```python
from build123d import *

# Parameters (mm, degrees)
BOSS_EXTRUDE1_DEPTH   = 227
CUT_EXTRUDE1_DEPTH    = 257.229581821
SKETCH3_W             = 10
SKETCH3_H             = 15.5
CUT_EXTRUDE2_DEPTH    = 234.473879022
SKETCH4_W             = 15.5
SKETCH4_H             = 10
CUT_EXTRUDE3_DEPTH    = 252.639093083
FILLET3_R             = 1.5
BOSS_EXTRUDE3_DEPTH   = 1.5
BOSS_EXTRUDE4_DEPTH   = 1.5
SKETCH9_W             = 26
SKETCH9_H             = 12
BOSS_EXTRUDE5_DEPTH   = 1.5
SKETCH10_W            = 12
SKETCH10_H            = 26
BOSS_EXTRUDE6_DEPTH   = 1.5
FILLET7_R             = 5
SKETCH11_R            = 2
CUT_EXTRUDE4_DEPTH    = 10
SKETCH12_R            = 2
CUT_EXTRUDE5_DEPTH    = 10
FILLET8_R             = 0.2
F_3_0MM_DOWEL_HOLE1_D = 3
F_3_0MM_DOWEL_HOLE2_D = 3


with BuildPart() as part:
    # Sketch1 → Boss-Extrude1 (new body)
    with BuildSketch(Plane.XY):
        Polygon((5.710530524, 107.230570717), (35.710530524, 107.230570717), (35.710530524, 97.694605712), (39.660530524, 97.694605712), (42.571762587, 100.605837775), (44.621762586, 98.555837776), (41.710530523, 95.644605712), (41.710530523, 91.694605712), (51.246495528, 91.694605712), (51.246495528, 61.694605712), align=None)
    extrude(amount=BOSS_EXTRUDE1_DEPTH)

    # Sketch2 → Cut-Extrude1 (cut, through all)
    with BuildSketch(Plane(origin=(0, 0, 0), x_dir=(-1, 0, 0), z_dir=(0, 0, -1))):
        Polygon((-45.246495528, 88.994605712), (-45.246495528, 80.994605712), (-43.746495528, 80.994605712), (-43.746495528, 88.994605712), (-39.660530524, 88.994605712), (-33.010530524, 95.644605712), (-33.010530524, 99.730570717), (-25.010530524, 99.730570717), (-25.010530524, 101.230570717), (-33.010530524, 101.230570717), (-33.010530524, 106.694605712), (-36.710530524, 106.694605712), (-36.710530524, 108.694605712), (27.289469476, 108.694605712), (-52.710530523, 28.694605712), (-52.710530523, 92.694605712), (-50.710530523, 92.694605712), (-50.710530523, 88.994605712), align=None)
    extrude(amount=-CUT_EXTRUDE1_DEPTH, mode=Mode.SUBTRACT)

    # Sketch3 → Cut-Extrude2 (cut, through all)
    with BuildSketch(Plane(origin=(0, 101.230570717, 0), x_dir=(1, 0, 0), z_dir=(0, 1, 0))):
        with Locations((28.010530524, -5.75)):
            Rectangle(SKETCH3_W, SKETCH3_H)
        with Locations((28.010530524, -221.25)):
            Rectangle(SKETCH3_W, SKETCH3_H)
        with BuildLine():
            Line((31.010530524, -28.5), (31.010530524, -198.5))
            ThreePointArc((31.010530524, -198.5), (29.010530524, -200.5), (27.010530524, -198.5))
            Line((27.010530524, -198.5), (27.010530524, -28.5))
            ThreePointArc((27.010530524, -28.5), (29.010530524, -26.5), (31.010530524, -28.5))
        make_face()
    extrude(amount=-CUT_EXTRUDE2_DEPTH, mode=Mode.SUBTRACT)

    # Sketch4 → Cut-Extrude3 (cut, through all)
    with BuildSketch(Plane(origin=(45.246495528, 0, 0), x_dir=(0, 0, -1), z_dir=(1, 0, 0))):
        with Locations((-221.25, 83.994605712)):
            Rectangle(SKETCH4_W, SKETCH4_H)
        with Locations((-5.75, 83.994605712)):
            Rectangle(SKETCH4_W, SKETCH4_H)
        with BuildLine():
            Line((-198.5, 86.994605712), (-28.5, 86.994605712))
            ThreePointArc((-28.5, 86.994605712), (-26.5, 84.994605712), (-28.5, 82.994605712))
            Line((-28.5, 82.994605712), (-198.5, 82.994605712))
            ThreePointArc((-198.5, 82.994605712), (-200.5, 84.994605712), (-198.5, 86.994605712))
        make_face()
    extrude(amount=-CUT_EXTRUDE3_DEPTH, mode=Mode.SUBTRACT)

    # Fillet3
    # the kernel refuses this fillet: 1.5 mm, written as the material it takes off along each edge
    with BuildSketch(Plane(origin=(44.621762586, 98.555837776, -3.75), x_dir=(-0.7071067811865522, -0.7071067811865428, 0), z_dir=(0, 0, 1)), Plane(origin=(42.571762587, 100.605837775, -3.75), x_dir=(0.7071067811865476, -0.7071067811865476, 0), z_dir=(0, 0, 1))) as fillet3_piece_1:
        with BuildLine():
            CenterArc((FILLET3_R, -FILLET3_R), FILLET3_R, 90, 90)
            Line((0, -FILLET3_R), (0, 0))
            Line((0, 0), (FILLET3_R, 0))
        make_face()
    extrude(amount=234.5, mode=Mode.SUBTRACT)

    # Sketch6 → Boss-Extrude3 (add)
    with BuildSketch(Plane(origin=(0, 0, 13.5), x_dir=(-1, 0, 0), z_dir=(0, 0, -1))):
        Polygon((-45.246495528, 90.194605712), (-45.246495528, 65.230570717), (-33.246495528, 65.230570717), (-33.246495528, 89.230570717), (-9.246495528, 89.230570717), (-9.246495528, 101.230570717), (-34.210530524, 101.230570717), (-34.210530524, 96.230570717), (-40.246495528, 90.194605712), align=None)
    extrude(amount=BOSS_EXTRUDE3_DEPTH)

    # Sketch7 → Boss-Extrude4 (add)
    with BuildSketch(Plane.XY.offset(213.5)):
        Polygon((9.246495528, 101.230570717), (34.210530524, 101.230570717), (34.210530524, 96.230570717), (40.246495528, 90.194605712), (45.246495528, 90.194605712), (45.246495528, 65.230570717), (33.246495528, 65.230570717), (33.246495528, 89.230570717), (9.246495528, 89.230570717), align=None)
    extrude(amount=BOSS_EXTRUDE4_DEPTH)

    # Sketch9 → Boss-Extrude5 (add)
    with BuildSketch(Plane(origin=(0, 101.230570717, 0), x_dir=(1, 0, 0), z_dir=(0, 1, 0))):
        with Locations((22.246495528, -209)):
            Rectangle(SKETCH9_W, SKETCH9_H)
        with Locations((22.246495528, -18)):
            Rectangle(SKETCH9_W, SKETCH9_H)
    extrude(amount=-BOSS_EXTRUDE5_DEPTH)

    # Sketch10 → Boss-Extrude6 (add)
    with BuildSketch(Plane(origin=(45.246495528, 0, 0), x_dir=(0, 0, -1), z_dir=(1, 0, 0))):
        with Locations((-209, 78.230570717)):
            Rectangle(SKETCH10_W, SKETCH10_H)
        with Locations((-18, 78.230570717)):
            Rectangle(SKETCH10_W, SKETCH10_H)
    extrude(amount=-BOSS_EXTRUDE6_DEPTH)

    # Fillet7
    fillet7_edges = [part.edges().sort_by_distance(p)[0] for p in [
        (33.246495528, 65.230570717, 12.75),
        (33.246495528, 89.230570717, 12.75),
        (9.246495528, 89.230570717, 12.75),
        (9.246495528, 89.230570717, 214.25),
        (33.246495528, 89.230570717, 214.25),
        (33.246495528, 65.230570717, 214.25),
        (9.246495528, 100.480570717, 203),
        (25.010530524, 100.480570717, 203),
        (9.246495528, 100.480570717, 24),
        (25.010530524, 100.480570717, 24),
        (44.496495528, 65.230570717, 203),
        (44.496495528, 80.994605712, 203),
        (44.496495528, 65.230570717, 24),
        (44.496495528, 80.994605712, 24),
    ]]
    fillet(fillet7_edges, radius=FILLET7_R)

    # Sketch11 → Cut-Extrude4 (cut)
    with BuildSketch(Plane(origin=(45.246495528, 0, 0), x_dir=(0, 0, -1), z_dir=(1, 0, 0))):
        with Locations(Location((-209.5, 84.994605712, 0), (0, 0, 90))):
            Circle(SKETCH11_R)
        with Locations(Location((-17.5, 84.994605712, 0), (0, 0, 90))):
            Circle(SKETCH11_R)
    extrude(amount=-CUT_EXTRUDE4_DEPTH, mode=Mode.SUBTRACT)

    # Sketch12 → Cut-Extrude5 (cut)
    with BuildSketch(Plane(origin=(0, 101.230570717, 0), x_dir=(1, 0, 0), z_dir=(0, 1, 0))):
        with Locations(Location((29.010530524, -17.5, 0), (0, 0, 270))):
            Circle(SKETCH12_R)
        with Locations(Location((29.010530524, -209.5, 0), (0, 0, 270))):
            Circle(SKETCH12_R)
    extrude(amount=-CUT_EXTRUDE5_DEPTH, mode=Mode.SUBTRACT)

    # Fillet8
    fillet8_edges = [part.edges().sort_by_distance(p)[0] for p in [
        (35.710530524, 97.694605712, 113.5),
        (39.660530524, 97.694605712, 113.5),
        (41.710530523, 95.644605712, 113.5),
        (41.710530523, 91.694605712, 113.5),
        (50.710530523, 91.694605712, 113.5),
        (35.710530524, 106.694605712, 113.5),
        (33.010530524, 106.694605712, 113.5),
        (50.710530523, 88.994605712, 113.5),
    ]]
    fillet(fillet8_edges, radius=FILLET8_R)

    # Ø3.0mm Dowel Hole1 (through all)
    with Locations(Plane.XY.offset(215)):
        with Locations((16.410530524, 93.494605712)):
            Hole(F_3_0MM_DOWEL_HOLE1_D / 2)

    # Ø3.0mm Dowel Hole2 (through all)
    with Locations(Plane.XY.offset(215)):
        with Locations((37.510530524, 72.394605712)):
            Hole(F_3_0MM_DOWEL_HOLE2_D / 2)


solid = part.part
```
Read the model definition and answer for the solid it produces. Units are mm, in the model's axes. A direction names the side the tool comes from. Coordinates: 2 decimals unless noted, no trailing zeros. Return JSON: item names as keys, results as strings.
1. Find the intervals of material crossed by line 1 along Z through (x, y) = (39, 69); line 2 along X through (y, z) = (101, 185); line 3 along Y through (x, z) = (41.5, 57), in increasing order. Write a range as from..to.
Found:
{"line 1": "12..13.5, 213.5..215", "line 2": "25.01..27.01, 31.01..35.71", "line 3": "88.99..99.53"}
2. A cutting plane is placed at A-A (z = 61.5). Give the number of separate pieces and of enclosed holes in the cut face, and give its area (3 significant figures).
Found:
{"separate pieces": "3", "enclosed holes": "0", "area": "123 mm2"}
3. Each of these flat-tipped pins is pushed along its axis until it touches: P1, Ø1.5, axis at y = 84, z = 176, coming from the -X side; P2, Ø1, axis at y = 83, z = 126, coming from the +X side; P3, Ø0.8, axis at x = 23, z = 214, coming from the -Y side; P4, Ø4, axis at y = 88.5, z = 98.5, coming from the +X side. Where does it stop, or does it pass through?
Found:
{"P1": "through", "P2": "x = 45.25", "P3": "y = 89.23", "P4": "x = 50.71"}
4. A tool of negligible diameter and unlimited length cuts with its end or side. For faces 1 (the face through (31, 90, 213.5)), 2 (the face through (23.51, 100.49, 201.57)), 3 (the face through (44.49, 66.66, 22.5)), 4 (the face through (41.711, 94, 112)), from which of +Z, -Z, +X, -X, +Y, -Y can it reach the whole face along a straight path? Write none if from no direction.
Found:
{"face 1": "-X, -Y", "face 2": "-X, +Y, -Y", "face 3": "+X, -X, -Y", "face 4": "+Z, -Z, +X"}
5. Determine the mould class of faces 5 (the face through (35.711, 102, 112)), 6 (the face through (42, 88.995, 112)), 7 (the face through (46, 91.695, 112)) for opening direction Y: pulls with the +Y half, pulls with the -Y half, needs draft (parallel to the pull), parting line crosses it, or undercut.
Found:
{"face 5": "needs draft", "face 6": "pulls with the -Y half", "face 7": "undercut"}
